For this review, take the finished solid that the model builds, in its own axes (mm). Coordinates: 2 decimals unless noted, no trailing zeros. Write each loop counter-clockwise with the first axis right and the second up, starting at its lowest first coordinate (ties: lowest second). Pieces come first, ordered by that corner, then holes.
```python
from build123d import *

# Parameters (mm, degrees)
F1_DEPTH = 25
F2_R     = 0.5


with BuildPart() as f1:
    # F0 (on Front) → F1 (new body)
    with BuildSketch(Plane.XZ):
        with BuildLine():
            Line((25, 0), (11, 41))
            ThreePointArc((11, 41), (0, 30), (-11, 41))
            Line((-11, 41), (-25, 0))
            Line((-25, 0), (25, 0))
        make_face()
    extrude(amount=F1_DEPTH)

    # F2
    f2_edges = [f1.edges().sort_by_distance(p)[0] for p in [
        (-11, -12.5, 41),
        (11, -12.5, 41),
    ]]
    fillet(f2_edges, radius=F2_R)


solid = f1.part
```
1) The part is to be moulded in two halves that separate along X. For faces 1 (the face through (0, 0, 16)), 2 (the face through (0, -12, 30)), 3 (the face through (-18.276, -12.325, 19.693)), say which applies: pulls with the +X half, pulls with the -X half, needs draft (parallel to the pull), parting line crosses it, or undercut.
2) For L1, parallel to X at y = -5.25, z = 37; L2, parallel to X at y = -21.5, z = 36; L3, parallel to X at y = -9.25, z = 11, list the stretches that pass through material, from the lowest coordinate up.
3) Consider section D-D (z = 22). Give the boundary of the cut face in (x, y), then the cut area to 3 significant figures.
4) Consider section C-C (x = 16). Give the boundary of the cut face in (y, z), then the cut area to 3 significant figures.
5) Clearance check with flat-ended pins moving along their axes: P1, Ø2, axis at x = 12.5, y = -7.5, coming from the +Z side; P2, Ø4, axis at y = -21, z = 30, coming from the -X side; P3, Ø8, axis at y = -16.5, z = 9, coming from the +X side. State where each tip first meets the part, or that it passes through.
6) Consider section A-A (y = -6.5). Give the boundary of the cut face in (x, z).
7) Consider section B-B (z = 34). Give the boundary of the cut face in (x, y).
Results:
1. face 1: needs draft
1. face 2: undercut
1. face 3: pulls with the -X half
2. L1: x = -12.37 to -10.25, 10.25 to 12.37
2. L2: x = -12.71 to -9.8, 9.8 to 12.71
2. L3: x = -21.24 to 21.24
3. outline: (-17.49, -25) - (17.49, -25) - (17.49, 0) - (-17.49, 0) - close
3. area: 874 mm2
4. outline: (-25, 0) - (0, 0) - (0, 26.36) - (-25, 26.36) - close
4. area: 659 mm2
5. P1: stops at z = 39.12
5. P2: stops at x = -15.44
5. P3: stops at x = 23.29
6. outline: (-25, 0) - (25, 0) - (11.74, 38.84) arc R0.5 ccw to (10.77, 38.78) arc R11 cw to (-10.77, 38.78) arc R0.5 ccw to (-11.74, 38.84) - close
7. outline: (-13.39, -25) - (-8.49, -25) - (-8.49, 0) - (-13.39, 0) - close; (8.49, -25) - (13.39, -25) - (13.39, 0) - (8.49, 0) - close
